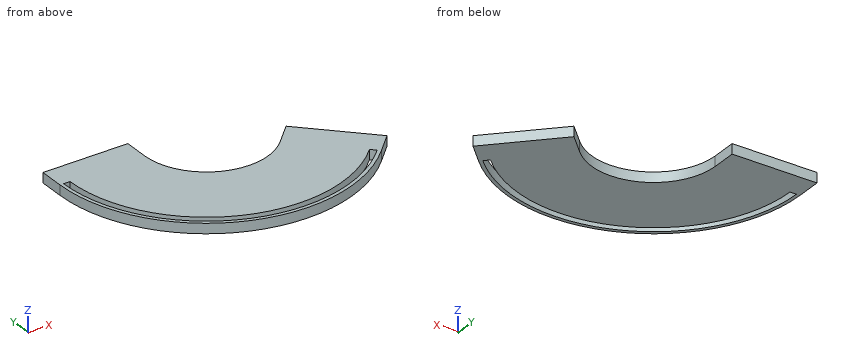
```python
from build123d import *

# Parameters (mm, degrees)
BOSS_EXTRUDE3_DEPTH = 5.08
CUT_EXTRUDE1_DEPTH  = 106.587982078


with BuildPart() as part:
    # Sketch2 → Boss-Extrude3 (new body)
    with BuildSketch(Plane.XY):
        with BuildLine():
            Line((22.537725188, -22.001112684), (31.517981309, -13.020856563))
            Line((31.517981309, -13.020856563), (61.981075074, -43.483950327))
            Line((61.981075074, -43.483950327), (53.000818953, -52.464206448))
            ThreePointArc((53.000818953, -52.464206448), (-28.188071212, -69.043554437), (-74.575034639, -0.379442341))
            Line((-74.575034639, -0.379442341), (-74.575034639, 12.320557659))
            Line((-74.575034639, 12.320557659), (-31.493714286, 12.320557659))
            Line((-31.493714286, 12.320557659), (-31.493714286, -0.379442341))
            ThreePointArc((-31.493714286, -0.379442341), (-11.701563668, -29.241604329), (22.537725188, -22.001112684))
        make_face()
    extrude(amount=BOSS_EXTRUDE3_DEPTH)

    # Sketch3 → Cut-Extrude1 (cut, through all)
    with BuildSketch(Plane.XY.offset(5.08)):
        with BuildLine():
            Line((-72.797011063, -0.379442341), (-69.494964077, -0.379442341))
            ThreePointArc((-69.494964077, -0.379442341), (-26.244012372, -64.35018122), (49.408666609, -48.872054105))
            Line((49.408666609, -48.872054105), (51.743566425, -51.20695392))
            ThreePointArc((51.743566425, -51.20695392), (-27.507651047, -67.400874846), (-72.797011063, -0.379442341))
        make_face()
    extrude(amount=-CUT_EXTRUDE1_DEPTH, mode=Mode.SUBTRACT)


solid = part.part
```
Here's how the part is built. I have some questions about the finished solid (model axes, mm). Coordinates: 2 decimals unless noted, no trailing zeros. Order: outer loops, then holes, each group sorted by start corner. A loop starts at its lowest first (then second) coordinate and runs counter-clockwise, first axis right, second up. Notation, with made-up numbers: M -26.5,62.25 L 20.5,62.25 A22 cw 20.5,70.25 Z; hole C 36,-31 d3. An arc over 180 degrees is marked long. Answer as a JSON object with one key per item and string values. Group by question number.
(1) I need wall thicknesses on probe 1 along X at (y, z) = (-55, 4.45); probe 2 along X at (y, z) = (-54, 3.45); probe 3 along X at (y, z) = (4, 1.8). Which ranges of each line are inside material? Lowest first, please.
(2) Suppose I cut it at A-A, the plane x = 0. Please give me the cut outline in (y, z).
(3) For pin 1 (1.5 mm diameter, centred on y = 3.5, z = 3, fed in from +X); pin 2 (3 mm diameter, centred on y = -64, z = 2, fed in from +X); pin 3 (2 mm diameter, centred on x = 46.5, z = 1.5, fed in from -Y), each with a flat end and sliding along its axis, tell me the tip position at first contact or that it passes through.
(4) Suppose I cut it at B-B, the plane y = -54.5. Please give me the cut outline in (x, z), then the cut area to 3 significant figures.
(5) Suppose I cut it at C-C, the plane z = 3.45. Please give me the cut outline in (x, y).
(6) Suppose I cut it at D-D, the plane y = -9. Please give me the cut outline in (x, z), then the cut area to 3 significant figures.
Values found:
{
 "1": {"probe 1": "x = -50.36 to -47.69, -42.48 to 42.48, 47.69 to 50.36", "probe 2": "x = -51.44 to -48.82, -43.75 to 43.75, 48.82 to 51.44", "probe 3": "x = -74.58 to -31.49"},
 "2": {"outline": "M -74.58,0 L -72.8,0 L -72.8,5.08 L -74.58,5.08 Z; M -69.5,0 L -31.5,0 L -31.5,5.08 L -69.5,5.08 Z"},
 "3": {"pin 1": "stops at x = -31.49", "pin 2": "stops at x = 40.69", "pin 3": "stops at y = -59.09"},
 "4": {"outline": "M -50.91,0 L -48.26,0 L -48.26,5.08 L -50.91,5.08 Z; M -43.12,0 L 43.12,0 L 43.12,5.08 L -43.12,5.08 Z; M 48.26,0 L 50.91,0 L 50.91,5.08 L 48.26,5.08 Z", "area": "465 mm^2"},
 "5": {"outline": "M -74.58,-0.38 A74.58 ccw 53,-52.46 L 61.98,-43.48 L 31.52,-13.02 L 22.54,-22 A31.5 cw -31.49,-0.38 L -31.49,12.32 L -74.58,12.32 Z; hole M -72.8,-0.38 A72.8 ccw 51.74,-51.21 L 49.41,-48.87 A69.5 cw -69.49,-0.38 Z"},
 "6": {"outline": "M -74.03,0 L -72.24,0 L -72.24,5.08 L -74.03,5.08 Z; M -68.91,0 L -30.18,0 L -30.18,5.08 L -68.91,5.08 Z", "area": "206 mm^2"}
}
